Geometry check sheet. Reference: the model listing, model coordinates, mm. A direction names the side the tool comes from. Give positions to 0.01 mm unless a question says otherwise; leave off trailing zeros. Write each loop counter-clockwise with the first axis right and the second up, starting at its lowest first coordinate (ties: lowest second). Pieces come first, ordered by that corner, then holes. Notation, with made-up numbers: M 83.25,63.5 L 96.25,63.5 A28 cw 96.25,100.5 Z; hole C 87.25,43.5 d9. An arc over 180 degrees is marked long. Write each question's results on one line, items separated by ' | '.
```python
from build123d import *

# Parameters (mm, degrees)
SKETCH7_R               = 5.5
SKETCH7_R_2             = 28
MAIN_BODY_DEPTH         = 30
BOLT_HEAD_COUNTERSINK_R = 9.5
COUNTERSINK_HOLES_DEPTH = 11
SKETCH9_R               = 32.45
CUT_EXTRUDE2_DEPTH      = 26
CUT_EXTRUDE3_DEPTH      = 15
ROUND_EDGES_R           = 3
F_30_CHAMFER1_SIZE      = 1.5
F_30_CHAMFER1_SIZE2     = 0.866025404
SKETCH11_R              = 44.5
SKETCH11_R_2            = 38.5
SKETCH11_R_3            = 17.5
SKETCH11_R_4            = 11.5
SKETCH11_R_5            = 14
SKETCH11_R_6            = 8
CUT_EXTRUDE4_DEPTH      = 3


with BuildPart() as part:
    # Sketch7 → Main body (new body)
    with BuildSketch(Plane(origin=(0, 0, 0), x_dir=(1, 0, 0), z_dir=(0, 1, 0))):
        with BuildLine():
            Line((-91.813057025, -8.005811355), (-84.980564836, -80.685361783))
            ThreePointArc((-84.980564836, -80.685361783), (-80.697244338, -88.79601226), (-71.936363988, -91.511976387))
            Line((-71.936363988, -91.511976387), (87.393822743, -76.886943186))
            ThreePointArc((87.393822743, -76.886943186), (95.514657683, -72.620523346), (98.248872823, -63.864133341))
            Line((98.248872823, -63.864133341), (89.6645061, 31.751287215))
            ThreePointArc((89.6645061, 31.751287215), (81.254432476, 42.143635856), (68.448272489, 38.305340008))
            ThreePointArc((68.448272489, 38.305340008), (65.405823358, 35.822809296), (61.642082029, 34.703118865))
            Line((61.642082029, 34.703118865), (40.782608291, 32.788412667))
            ThreePointArc((40.782608291, 32.788412667), (36.543989689, 33.315359566), (32.911888119, 35.562891293))
            ThreePointArc((32.911888119, 35.562891293), (4.765471685, 48.687341482), (-25.474547855, 41.615342543))
            Line((-25.474547855, 41.615342543), (-86.26800446, 3.266768015))
            ThreePointArc((-86.26800446, 3.266768015), (-90.633494009, -1.585933038), (-91.813057025, -8.005811355))
        make_face()
        with Locations(Location((77.712578531, 30.678241374, 0), (0, 0, 270))):
            Circle(SKETCH7_R, mode=Mode.SUBTRACT)
        with Locations(Location((-79.865733667, -6.882661954, 0), (0, 0, 270))):
            Circle(SKETCH7_R, mode=Mode.SUBTRACT)
        with Locations(Location((86.296945253, -64.937179181, 0), (0, 0, 270))):
            Circle(SKETCH7_R, mode=Mode.SUBTRACT)
        with Locations(Location((-73.033241478, -79.562212382, 0), (0, 0, 270))):
            Circle(SKETCH7_R, mode=Mode.SUBTRACT)
        with Locations(Location((-0.132225968, 1.440515582, 0), (0, 0, 270))):
            Circle(SKETCH7_R_2, mode=Mode.SUBTRACT)
    extrude(amount=MAIN_BODY_DEPTH)

    # bolt head countersink → countersink holes (cut)
    with BuildSketch(Plane(origin=(0, 30, 0), x_dir=(1, 0, 0), z_dir=(0, 1, 0))):
        with Locations(Location((-79.865733667, -6.882661954, 0), (0, 0, 270))):
            Circle(BOLT_HEAD_COUNTERSINK_R)
        with Locations(Location((-73.033241478, -79.562212382, 0), (0, 0, 270))):
            Circle(BOLT_HEAD_COUNTERSINK_R)
        with Locations(Location((77.712578531, 30.678241374, 0), (0, 0, 270))):
            Circle(BOLT_HEAD_COUNTERSINK_R)
        with Locations(Location((86.296945253, -64.937179181, 0), (0, 0, 270))):
            Circle(BOLT_HEAD_COUNTERSINK_R)
    extrude(amount=-COUNTERSINK_HOLES_DEPTH, mode=Mode.SUBTRACT)

    # Sketch9 → Cut-Extrude2 (cut)
    with BuildSketch(Plane(origin=(0, 30, 0), x_dir=(1, 0, 0), z_dir=(0, 1, 0))):
        with Locations(Location((-0.132225968, 1.440515582, 0), (0, 0, 270))):
            Circle(SKETCH9_R)
    extrude(amount=-CUT_EXTRUDE2_DEPTH, mode=Mode.SUBTRACT)

    # Sketch10 → Cut-Extrude3 (cut)
    with BuildSketch(Plane(origin=(0, 30, 0), x_dir=(1, 0, 0), z_dir=(0, 1, 0))):
        with BuildLine():
            Line((-46.230998709, 66.050698395), (-40.039175854, -1.286268383))
            ThreePointArc((-40.039175854, -1.286268383), (3.059511975, -38.431941189), (39.700320715, 5.096773882))
            Line((39.700320715, 5.096773882), (33.434094657, 73.363214995))
            Line((33.434094657, 73.363214995), (-46.230998709, 66.050698395))
        make_face()
    extrude(amount=-CUT_EXTRUDE3_DEPTH, mode=Mode.SUBTRACT)

    # round edges
    round_edges_edges = [part.edges().sort_by_distance(p)[0] for p in [
        (-42.96933308, 22.5, -30.579614152),
        (37.127163098, 22.5, -33.12964587),
    ]]
    fillet(round_edges_edges, radius=ROUND_EDGES_R)

    # 30 Chamfer1
    f_30_chamfer1_edges = [part.edges().sort_by_distance(p)[0] for p in [
        (-0.132225968, 15, -33.890515582),
    ]]
    f_30_chamfer1_side = [part.faces().sort_by_distance(p)[0] for p in [
        (-0.132225968, 9.5, -33.890515582),
    ]]
    chamfer(f_30_chamfer1_edges, length=F_30_CHAMFER1_SIZE, length2=F_30_CHAMFER1_SIZE2, reference=f_30_chamfer1_side[0])

    # Sketch11 → Cut-Extrude4 (cut)
    # profile 1 of 3: a face of its own
    with BuildSketch(Plane.XZ):
        with Locations(Location((-0.132225968, -1.440515582, 0), (0, 0, 270))):
            Circle(SKETCH11_R)
        with Locations(Location((-0.132225968, -1.440515582, 0), (0, 0, 270))):
            Circle(SKETCH11_R_2, mode=Mode.SUBTRACT)
    # profile 2 of 3: a face of its own
    with BuildSketch(Plane.XZ):
        with Locations(Location((-54.514942776, 62.86283352, 0), (0, 0, 270))):
            Circle(SKETCH11_R_3)
        with Locations(Location((-54.514942776, 62.86283352, 0), (0, 0, 270))):
            Circle(SKETCH11_R_4, mode=Mode.SUBTRACT)
    # profile 3 of 3: a face of its own
    with BuildSketch(Plane.XZ):
        with Locations(Location((67.139628144, 30.48677163, 0), (0, 0, 270))):
            Circle(SKETCH11_R_5)
        with Locations(Location((67.139628144, 30.48677163, 0), (0, 0, 270))):
            Circle(SKETCH11_R_6, mode=Mode.SUBTRACT)
    extrude(amount=-CUT_EXTRUDE4_DEPTH, mode=Mode.SUBTRACT)


solid = part.part
```
Q1. Material ranges on probe 1 along X at (y, z) = (25, 10.5); probe 2 along Z at (x, y) = (22.5, 8); probe 3 along Z at (x, y) = (-77, 13.75), recorded low to high. Write a range as [from, to].
Answer key:
probe 1: x = [-91.58, -88.65], [-71.08, -38.31], [38.04, 93.46] | probe 2: z = [-43.2, -24.7], [21.81, 82.84] | probe 3: z = [-9.11, 2.19], [11.58, 75.75], [83.37, 90.89]
Q2. Access from +Z, -Z, +X, -X, +Y, -Y to the whole of each face (thin tool, end or side, straight path). Record for faces 4 (the face through (36.601, 8.123, -33.295)), 5 (the face through (-41.298, 22.605, -12.399)), 6 (the face through (61, 3, 24)), 7 (the face through (21.799, 8.817, -25.358)), 8 (the face through (2, 0, 52)).
Answer key:
face 4: -Z, +Y, -Y | face 5: -Z, +Y | face 6: -Y | face 7: +Y | face 8: +Z, -Z, +X, -X, -Y
Q3. Depth check by flat-ended pin: P1, Ø2, axis at y = 14.5, z = 69, coming from the +X side; P2, Ø11.5, axis at x = -73.03, z = 79.56, coming from the +Y side; P3, Ø21, axis at x = 75, z = -27.5, coming from the +Y side; P4, Ø9, axis at x = -73.03, z = 79.56, coming from the -Y side. Enter the tip coordinate at first touch or a pass-through.
Answer key:
P1: stops at x = 97.9 | P2: stops at y = 19 | P3: stops at y = 30 | P4: passes through
Q4. Section check A-A (y = 23.5). Enter the section's corners in (x, z).
Answer key:
outline: M -91.81,8.01 A12 ccw -86.27,-3.27 L -47.11,-27.97 A3 ccw -42.52,-25.71 L -40.04,1.29 A40 cw long 39.7,-5.1 L 37.46,-29.49 A3 ccw 40.32,-32.76 A10 cw 40.78,-32.79 L 61.64,-34.7 A10 cw 68.45,-38.31 A12 ccw 89.66,-31.75 L 98.25,63.86 A12 ccw 87.39,76.89 L -71.94,91.51 A12 ccw -84.98,80.69 Z; hole C -79.87,6.88 d19; hole C -73.03,79.56 d19; hole C 77.71,-30.68 d19; hole C 86.3,64.94 d19
Q5. Release check for a two-part mould opening along Z. For faces 1 (the face through (-14, 4, -26)), 2 (the face through (65.455, 14.79, -35.849)), 3 (the face through (-80.8, 14.79, 88.71)) record: released by +Z, released by -Z, zero draft, split by the parting line, or undercut.
Answer key:
face 1: undercut | face 2: released by -Z | face 3: released by +Z
